Work out the finished part from the listing and answer in its coordinate system (mm). Face numbers are marked on the shaded views. A direction names the side the tool comes from. Round coordinates to 2 decimals unless told otherwise and drop trailing zeros. Loops run counter-clockwise (first coordinate to the right, second up) from the corner with the lowest first, then second, coordinate; pieces in that order, holes last. Notation, with made-up numbers: M 22,62.5 L 44,62.5 A21 ccw 44,70.5 Z; hole C 57,68.25 d9. An arc over 180 degrees is marked long. One line per item, written item: value.
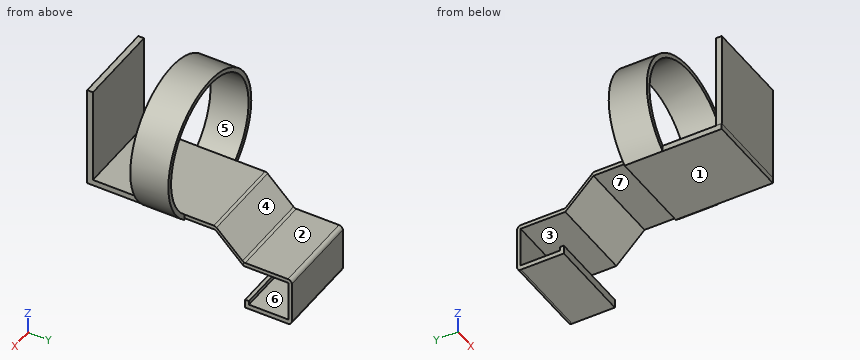
```python
from build123d import *

# Parameters (mm, degrees)
SKETCH2_W            = 55.901800272
SKETCH2_H            = 3.137316852
BOSS_EXTRUDE1_DEPTH  = 36.83
SKETCH3_W            = 55.901800272
SKETCH3_H            = 2.258710987
BOSS_EXTRUDE2_DEPTH  = 29.21
SKETCH4_W            = 55.901800272
SKETCH4_H            = 2.656475696
BOSS_EXTRUDE3_DEPTH  = 29.21
BOSS_EXTRUDE4_DEPTH  = 55.88
SKETCH7_W            = 55.88
SKETCH7_H            = 2.656475696
BOSS_EXTRUDE5_DEPTH  = 83.82
SKETCH8_W            = 55.88
SKETCH8_H            = 3.77839036
BOSS_EXTRUDE6_DEPTH  = 63.5
SKETCH18_W           = 55.901800272
SKETCH18_H           = 2.413327827
BOSS_EXTRUDE9_DEPTH  = 3.81
SKETCH20_R           = 45.365929921
BOSS_EXTRUDE10_DEPTH = 59.69
CUT_EXTRUDE2_DEPTH   = 59.69
CUT_EXTRUDE4_DEPTH   = 59.69
SKETCH23_R           = 50.619817538
CUT_EXTRUDE5_DEPTH   = 34.798
SKETCH24_W           = 55.992252849
SKETCH24_H           = 3.903032237
BOSS_EXTRUDE11_DEPTH = 38.608
SKETCH25_W           = 55.901800272
SKETCH25_H           = 6.947316852
CUT_EXTRUDE6_DEPTH   = 6.35
SKETCH26_W           = 55.901800272
SKETCH26_H           = 2.460794709
BOSS_EXTRUDE12_DEPTH = 2.54
FILLET2_R            = 2.54
FILLET4_R            = 2.54
FILLET5_R            = 2.54


with BuildPart() as part:
    # Sketch2 → Boss-Extrude1 (new body)
    with BuildSketch(Plane(origin=(0, 0, 0), x_dir=(1, 0, 0), z_dir=(0, 1, 0))):
        with Locations((27.950900136, 1.568658426)):
            Rectangle(SKETCH2_W, SKETCH2_H)
    extrude(amount=BOSS_EXTRUDE1_DEPTH)

    # Sketch3 → Boss-Extrude2 (add)
    with BuildSketch(Plane.XY):
        with Locations((27.950900136, 35.700644507)):
            Rectangle(SKETCH3_W, SKETCH3_H)
    extrude(amount=BOSS_EXTRUDE2_DEPTH)

    # Sketch4 → Boss-Extrude3 (add)
    with BuildSketch(Plane.XZ.offset(-34.571289013)):
        with Locations((27.950900136, 27.881762152)):
            Rectangle(SKETCH4_W, SKETCH4_H)
    extrude(amount=BOSS_EXTRUDE3_DEPTH)

    # Sketch6 → Boss-Extrude4 (add)
    with BuildSketch(Plane.ZY):
        Polygon((29.21, 5.361289013), (29.21, 8.93281191), (29.21, 36.83), (-3.137316852, 36.83), (-3.137316852, 0), (0, 0), (0, 34.571289013), (26.553524304, 34.571289013), (26.553524304, 5.361289013), (44.996482377, -13.08166906), (47.652958073, -13.08166906), align=None)
    extrude(amount=-BOSS_EXTRUDE4_DEPTH)

    # Sketch7 → Boss-Extrude5 (add)
    with BuildSketch(Plane.XZ.offset(13.08166906)):
        with Locations((27.94, 46.324720225)):
            Rectangle(SKETCH7_W, SKETCH7_H)
    extrude(amount=BOSS_EXTRUDE5_DEPTH)

    # Sketch8 → Boss-Extrude6 (add)
    with BuildSketch(Plane.XY.offset(47.652958073)):
        with Locations((27.94, -95.01247388)):
            Rectangle(SKETCH8_W, SKETCH8_H)
    extrude(amount=BOSS_EXTRUDE6_DEPTH)

    # Sketch18 → Boss-Extrude9 (add)
    with BuildSketch(Plane.XY):
        with Locations((27.950900136, 1.206663914)):
            Rectangle(SKETCH18_W, SKETCH18_H)
    extrude(amount=BOSS_EXTRUDE9_DEPTH)

    # Sketch20 → Boss-Extrude10 (add)
    with BuildSketch(Plane(origin=(0, -93.1232787, 0), x_dir=(1, 0, 0), z_dir=(0, 1, 0))):
        with Locations((27.94, -79.402958073)):
            Circle(SKETCH20_R)
    extrude(amount=BOSS_EXTRUDE10_DEPTH)

    # Sketch21 → Cut-Extrude2 (cut)
    with BuildSketch(Plane(origin=(0, -33.4332787, 0), x_dir=(1, 0, 0), z_dir=(0, 1, 0))):
        with BuildLine():
            Line((55.88, -47.652958073), (0, -47.652958073))
            ThreePointArc((0, -47.652958073), (27.94, -121.892938161), (55.88, -47.652958073))
        make_face()
    extrude(amount=-CUT_EXTRUDE2_DEPTH, mode=Mode.SUBTRACT)

    # Sketch22 → Cut-Extrude4 (cut)
    with BuildSketch(Plane(origin=(0, -33.4332787, 0), x_dir=(1, 0, 0), z_dir=(0, 1, 0))):
        Polygon((-0.112252849, -43.749925836), (55.992252849, -43.749925836), (52.485687981, -29.879615978), (-0.112252849, -30.827478948), align=None)
    extrude(amount=-CUT_EXTRUDE4_DEPTH, mode=Mode.SUBTRACT)

    # Sketch23 → Cut-Extrude5 (cut)
    with BuildSketch(Plane.XZ.offset(93.1232787)):
        with Locations((27.94, 84.259406915)):
            Circle(SKETCH23_R)
    extrude(amount=-CUT_EXTRUDE5_DEPTH, mode=Mode.SUBTRACT)

    # Sketch24 → Boss-Extrude11 (add)
    with BuildSketch(Plane.XZ.offset(58.3252787)):
        with Locations((27.883873576, 45.701441954)):
            Rectangle(SKETCH24_W, SKETCH24_H)
    extrude(amount=BOSS_EXTRUDE11_DEPTH)

    # Sketch25 → Cut-Extrude6 (cut)
    with BuildSketch(Plane.XZ):
        with Locations((27.950900136, 0.336341574)):
            Rectangle(SKETCH25_W, SKETCH25_H)
    extrude(amount=-CUT_EXTRUDE6_DEPTH, mode=Mode.SUBTRACT)

    # Sketch26 → Boss-Extrude12 (add)
    with BuildSketch(Plane.XY):
        with Locations((27.950900136, 7.580397355)):
            Rectangle(SKETCH26_W, SKETCH26_H)
    extrude(amount=BOSS_EXTRUDE12_DEPTH)

    # Fillet2
    fillet2_edges = [part.edges().sort_by_distance(p)[0] for p in [
        (27.950900136, 36.83, -3.137316852),
        (27.950900136, 36.83, 29.21),
    ]]
    fillet(fillet2_edges, radius=FILLET2_R)

    # Fillet4
    fillet4_edges = [part.edges().sort_by_distance(p)[0] for p in [
        (27.94, 5.361289013, 29.21),
    ]]
    fillet(fillet4_edges, radius=FILLET4_R)

    # Fillet5
    fillet5_edges = [part.edges().sort_by_distance(p)[0] for p in [
        (27.94, -13.08166906, 47.652958073),
    ]]
    fillet(fillet5_edges, radius=FILLET5_R)


solid = part.part
```
1) Find the intervals of material crossed by probe 1 along Z at (x, y) = (27.94, -49); probe 2 along Z at (x, y) = (31.5, 9.5); probe 3 along Z at (x, y) = (0.5, -89), in increasing order. Write a range as from..to.
Check values:
probe 1: 43.75..47.65, 121.89..124.77
probe 2: -3.14..0, 26.55..29.21
probe 3: 43.75..47.65
2) The mould has two halves that part along Y. Classify the marked faces 4, 5, 6 and 7: +Y half, -Y half, draft (parallel to the pull), parting line (faces both ways), or undercut.
Check values:
face 4: +Y half
face 5: draft
face 6: undercut
face 7: undercut
3) Find section B-B (y = -44.5). Give the vertices of the cut face in (x, z).
Check values:
outline: M -0.11,43.75 L 55.99,43.75 A45.37 ccw long Z; hole M 0,47.65 L 55.88,47.65 A42.38 ccw long Z
4) For the marked faces 1, 2 and 3, determine the directions among +Z, -Z, +X, -X, +Y, -Y from which every point of the face is accessible in a straight line to the end or side of a thin tool.
Check values:
face 1: -Z, +X, -X, -Y
face 2: +Z, +X, -X, +Y
face 3: +X, -X, -Y
5) Each of these flat-tipped pins is pushed along its axis until it touches: pin 1 (8 mm diameter, centred on y = -46, z = 55, fed in from +X); pin 2 (1.1 mm diameter, centred on y = -95.5, z = 67, fed in from -X); pin 3 (13 mm diameter, centred on x = 26, y = 15.5, fed in from +Z). Where does it stop, or does it pass through?
Check values:
pin 1: x = 68.46
pin 2: x = 0
pin 3: z = 29.21
6) Find section D-D (z = 34). Give the vertices of the cut face in (x, y).
Check values:
outline: M 0,-2.09 L 55.88,-2.09 L 55.88,0.57 L 0,0.57 Z
